Part model, mm, in its own coordinate system. Face numbers are marked on the shaded views. A direction names the side the tool comes from. Give positions to 0.01 mm unless a question says otherwise; leave off trailing zeros. Order: outer loops, then holes, each group sorted by start corner. A loop starts at its lowest first (then second) coordinate and runs counter-clockwise, first axis right, second up. Notation, with made-up numbers: (63, 17.5) -> (72, 17.5) arc R17 cw to (72, 28.5) -> close; hole circle Ø2 at (4.5, 66). An arc over 180 degrees is marked (long way). Write item = value, one per line. Start each with the question number.
Item 1: Tool access for the marked faces 4, 5, 6 and 7: list every direction of +Z, -Z, +X, -X, +Y, -Y with a clear straight run to the whole face (end or side of a thin tool).
Item 2: Flat gauge pins, fed straight in: P1, Ø6, axis at x = -26, z = 63.5, coming from the -Y side; P2, Ø3, axis at y = 8.05, z = 97.5, coming from the +X side; P3, Ø7, axis at x = 36.5, z = 43, coming from the +Y side. Where does each tip first touch, or does it go through?
Item 3: Drill centre lines: line 1 along Y through (x, z) = (17, 92); line 2 along Z through (x, y) = (40, 0); line 3 along Z through (x, y) = (-2.5, -10). Where is each one in solid material? Low to high.
Item 4: Band-saw the part on A-A on y = -0.5. Write the cut outline in (x, z).
Item 5: Pull direction Z, two halves, no side cores. Call the marked faces 1, 2 and 3: +Z half, -Z half, draft (parallel to the pull), parting line (faces both ways), or undercut.
```python
from build123d import *
from OCP.BRepAlgoAPI import BRepAlgoAPI_Cut
from OCP.TopTools import TopTools_ListOfShape

# Parameters (mm, degrees)
BOSS_EXTRUDE1_DEPTH = 140
SKETCH2_W           = 45
SKETCH2_H           = 25
SKETCH2_H_2         = 42
CUT_EXTRUDE1_DEPTH  = 151.712117272
SKETCH3_W           = 25
SKETCH3_H           = 58.39699261
SKETCH3_H_2         = 53.941763905
CUT_EXTRUDE2_DEPTH  = 149.913368614
CUT_EXTRUDE3_START  = -25
CUT_EXTRUDE3_DEPTH  = 25
SKETCH5_R           = 2.5
CUT_EXTRUDE4_DEPTH  = 128.82465442
SKETCH6_W           = 42
SKETCH6_H           = 41.970965134
CUT_EXTRUDE5_DEPTH  = 28
M3_TAPPED_HOLE1_D   = 2.5
CUT_EXTRUDE7_DEPTH  = 10
CUT_EXTRUDE8_DEPTH  = 10
CUT_EXTRUDE9_DEPTH  = 142.067055339


with BuildPart() as part:
    # Sketch1 → Boss-Extrude1 (new body)
    with BuildSketch(Plane.XY):
        with BuildLine():
            Line((-28.369303649, 18.31966037), (-28.369303649, -2.282608696))
            add(Edge.make_bspline(
                [(-28.369303649, -2.282608696), (2.684029018, -2.430944497), (-15.214915802, -21.968601645), (5.015839683, -23.456157195)],
                knots=[0, 0, 0, 0, 1, 1, 1, 1], degree=3))
            Line((5.015839683, -23.456157195), (49.891304348, -23.456157195))
            Line((49.891304348, -23.456157195), (49.891304348, -18.537678935))
            Line((49.891304348, -18.537678935), (14.347826087, -18.537678935))
            ThreePointArc((14.347826087, -18.537678935), (6.766304348, -10.956157195), (14.347826087, -3.374635456))
            Line((14.347826087, -3.374635456), (49.891304348, -3.374635456))
            Line((49.891304348, -3.374635456), (49.891304348, 1.543842805))
            Line((49.891304348, 1.543842805), (4.891304348, 1.543842805))
            add(Edge.make_bspline(
                [(-28.369303649, 18.31966037), (-6.165269931, 20.270771045), (-8.304675764, 7.778503855), (4.891304348, 1.543842805)],
                knots=[0, 0, 0, 0, 1, 1, 1, 1], degree=3))
        make_face()
    extrude(amount=BOSS_EXTRUDE1_DEPTH)

    # Sketch2 → Cut-Extrude1 (cut, through all)
    with BuildSketch(Plane(origin=(0, 1.543842805, 0), x_dir=(1, 0, 0), z_dir=(0, 1, 0))):
        with Locations((27.391304348, -12.5)):
            Rectangle(SKETCH2_W, SKETCH2_H)
        with Locations((27.391304348, -70)):
            Rectangle(SKETCH2_W, SKETCH2_H_2)
        with Locations((27.391304348, -127.5)):
            Rectangle(SKETCH2_W, SKETCH2_H)
    extrude(amount=-CUT_EXTRUDE1_DEPTH, mode=Mode.SUBTRACT)

    # Sketch3 → Cut-Extrude2 (cut, through all)
    with BuildSketch(Plane(origin=(4.891304348, 0, 0), x_dir=(0, 0, -1), z_dir=(1, 0, 0))):
        with Locations((-127.5, 5.751761195)):
            Rectangle(SKETCH3_W, SKETCH3_H)
        with Locations((-12.5, 3.524146843)):
            Rectangle(SKETCH3_W, SKETCH3_H_2)
    extrude(amount=-CUT_EXTRUDE2_DEPTH, mode=Mode.SUBTRACT)


with BuildPart() as cut_extrude3_tool:
    # Cut-Extrude3: read off the stored shape, not the designer's step
    # Cut-Extrude3 outline → Cut-Extrude3 (new body)
    with BuildSketch(Plane(origin=(0, 1.543842805, 0), x_dir=(1, 0, 0), z_dir=(0, 1, 0)).offset(CUT_EXTRUDE3_START)):
        with BuildLine():
            ThreePointArc((37.891304348, -91), (46.376584834, -94.514719112), (49.891302974, -103))
            Line((49.891302974, -103), (49.891304348, -91))
            Line((49.891304348, -91), (37.891304348, -91))
        make_face()
        with BuildLine():
            ThreePointArc((49.891302974, -103), (46.376583863, -111.48528186), (37.891301601, -115))
            Line((37.891301601, -115), (49.891304348, -115))
            Line((49.891304348, -115), (49.891302974, -103))
        make_face()
        with BuildLine():
            ThreePointArc((37.891303148, -25), (46.376585298, -28.514718201), (49.891304348, -37))
            Line((49.891304348, -37), (49.891304348, -25))
            Line((49.891304348, -25), (37.891303148, -25))
        make_face()
        with BuildLine():
            ThreePointArc((49.891304348, -37), (46.376585294, -45.485281802), (37.891303138, -49))
            Line((37.891303138, -49), (49.891304348, -49))
            Line((49.891304348, -49), (49.891304348, -37))
        make_face()
    extrude(amount=CUT_EXTRUDE3_DEPTH)


with BuildPart() as part_1:
    add(part.part)

    # Cut-Extrude3: cut by cut_extrude3_tool, with a tolerance
    cut_extrude3_stock = TopTools_ListOfShape()
    cut_extrude3_stock.Append(part_1.part.wrapped)
    cut_extrude3_tools = TopTools_ListOfShape()
    cut_extrude3_tools.Append(cut_extrude3_tool.part.wrapped)
    cut_extrude3_cut = BRepAlgoAPI_Cut()
    cut_extrude3_cut.SetArguments(cut_extrude3_stock)
    cut_extrude3_cut.SetTools(cut_extrude3_tools)
    cut_extrude3_cut.SetFuzzyValue(0.00001)
    cut_extrude3_cut.Build()
    add(Compound.cast(cut_extrude3_cut.Shape()).solids(), mode=Mode.REPLACE)

    # Sketch5 → Cut-Extrude4 (cut, through all)
    with BuildSketch(Plane(origin=(0, 1.543842805, 0), x_dir=(1, 0, 0), z_dir=(0, 1, 0))):
        with Locations(Location((37.891304348, -37, 0), (0, 0, 180))):
            Circle(SKETCH5_R)
        with Locations(Location((37.891302974, -103, 0), (0, 0, 180))):
            Circle(SKETCH5_R)
    extrude(amount=-CUT_EXTRUDE4_DEPTH, mode=Mode.SUBTRACT)

    # Sketch6 → Cut-Extrude5 (cut)
    with BuildSketch(Plane(origin=(4.891304348, 0, 0), x_dir=(0, 0, -1), z_dir=(1, 0, 0))):
        with Locations((-70, -2.461252543)):
            Rectangle(SKETCH6_W, SKETCH6_H)
    extrude(amount=-CUT_EXTRUDE5_DEPTH, mode=Mode.SUBTRACT)

    # M3 Tapped Hole1 (through all)
    with Locations(Plane(origin=(-28.369303649, 8.053562831, 42.5), x_dir=(0, -1, 0), z_dir=(-1, 0, 0))):
        with Locations((0, 0), (0, 55)):
            Hole(M3_TAPPED_HOLE1_D / 2)

    # Sketch10 → Cut-Extrude7 (cut)
    with BuildSketch(Plane(origin=(0, 0, 91), x_dir=(-1, 0, 0), z_dir=(0, 0, -1))):
        Polygon((-6.055554522, 4.543842805), (23.108695652, 4.543842805), (23.108695652, 21.156391706), (-12.385539101, 21.156391706), align=None)
    extrude(amount=-CUT_EXTRUDE7_DEPTH, mode=Mode.SUBTRACT)

    # Sketch12 → Cut-Extrude8 (cut)
    with BuildSketch(Plane.XY.offset(49)):
        Polygon((10.285273621, 4.543842805), (-23.108695652, 4.543842805), (-23.108695652, 23.852692611), (13.93451424, 23.852692611), align=None)
    extrude(amount=-CUT_EXTRUDE8_DEPTH, mode=Mode.SUBTRACT)

    # Sketch13 → Cut-Extrude9 (cut, through all)
    with BuildSketch(Plane.ZY.offset(28.369303649)):
        with BuildLine():
            Line((86.648776757, 1.525435208), (53.351223243, 1.525435208))
            ThreePointArc((53.351223243, 1.525435208), (50.522796118, 2.697008083), (49.351223243, 5.525435208))
            Line((49.351223243, 5.525435208), (49.351223243, 10.511616467))
            ThreePointArc((49.351223243, 10.511616467), (50.522796118, 13.340043592), (53.351223243, 14.511616467))
            Line((53.351223243, 14.511616467), (86.648776757, 14.511616467))
            ThreePointArc((86.648776757, 14.511616467), (89.477203882, 13.340043592), (90.648776757, 10.511616467))
            Line((90.648776757, 10.511616467), (90.648776757, 5.525435208))
            ThreePointArc((90.648776757, 5.525435208), (89.477203882, 2.697008083), (86.648776757, 1.525435208))
        make_face()
    extrude(amount=-CUT_EXTRUDE9_DEPTH, mode=Mode.SUBTRACT)


solid = part_1.part
```
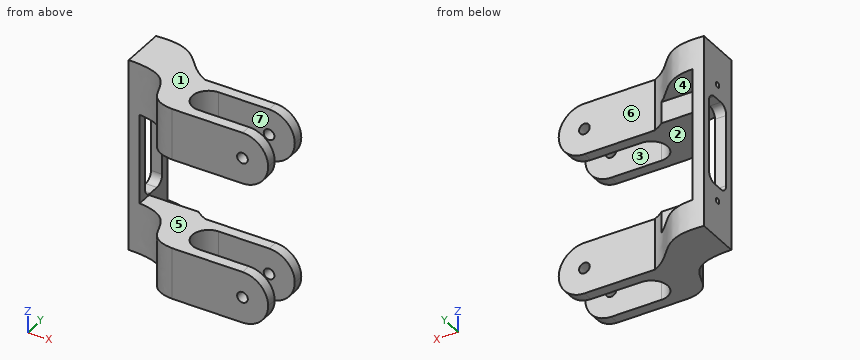
Values found:
q1.face_4 = +X, +Y
q1.face_5 = +X, +Y, -Y
q1.face_6 = +Z, -Z, +X, +Y
q1.face_7 = +Z, -Z, +X
q2.P1 = -2.53
q2.P2 = -23.11
q2.P3 = 1.54
q3.line_1 = -23.46 to -18.54, -3.37 to 1.54
q3.line_2 = 25.19 to 35.66, 38.34 to 48.81, 91.19 to 101.66, 104.34 to 114.81
q3.line_3 = 25 to 49, 91 to 115
q4.outline = (-28.37, 25) -> (37.89, 25) arc R12 ccw to (37.89, 49) -> (-23.11, 49) -> (-23.11, 91) -> (37.89, 91) arc R12 ccw to (37.89, 115) -> (-28.37, 115) -> close; hole circle Ø5 at (37.89, 37); hole circle Ø5 at (37.89, 103)
q5.face_1 = +Z half
q5.face_2 = undercut
q5.face_3 = draft
